Autodesk Inventor part; units mm, degrees
ref_plane "Płaszczyzna konstrukcyjna2" through (43, 47, -4.5) normal (0, 0, -1) x (-1, 0, 0)
ref_plane "YZ Plane" through (0, 0, 0) normal (1, 0, 0) x (0, 1, 0)
ref_plane "XZ Plane" through (0, 0, 0) normal (0, 1, 0) x (-1, 0, 0)
sketch "Szkic1" plane through (0, 0, 0) normal (0, 0, 1) x (1, 0, 0)
  line L0 (0, 0) -> (41, 0)
  line L1 (41, 0) -> (41, 45)
  line L2 (41, 45) -> (0, 45)
  line L3 (0, 45) -> (0, 0)
  line L4 (0, 45) -> (-2, 45)
  line L5 (-2, 45) -> (-2, 47)
  line L6 (41, 0) -> (41, -2)
  line L7 (41, -2) -> (43, -2)
  line L8 (43, -2) -> (-2, -2)
  line L9 (-2, -2) -> (-2, 47)
  line L10 (-2, 47) -> (43, 47)
  line L11 (43, 47) -> (43, -2)
  line L12 (41, 45) -> (37, 45)
  line L13 (37, 45) -> (37, 47)
  line L14 (43, 47) -> (37, 47)
  line L15 (41, 45) -> (41, 41)
  line L16 (41, 41) -> (43, 41)
  line L17 (43, 47) -> (43, 41)
  line L18 (43, 47) -> (37, 47)
  line L19 (20.5, 47) -> (20.5, -2)
  line L20 (-2, 22.5) -> (43, 22.5)
  line L21 (0, 45) -> (41, 45)
  line L22 (43, 47) -> (-2, 47)
  line L23 (-2, 47) -> (-2, -2)
  line L24 (4, 45) -> (4, 47)
  line L25 (0, 41) -> (-2, 41)
  line L26 (41, 0) -> (0, 0)
  line L27 (0, 0) -> (0, 45)
  line L28 (0, 0) -> (-2, 0)
  line L29 (-2, -2) -> (43, -2)
  line L30 (43, -2) -> (43, 47)
  line L31 (41, 4) -> (43, 4)
  line L32 (-2, -2) -> (-2, 47)
  line L33 (4, 0) -> (4, -2)
  line L34 (0, 0) -> (0, 4)
  line L35 (0, 4) -> (-2, 4)
  line L36 (41, 0) -> (37, 0)
  line L37 (37, 0) -> (37, -2)
  line L38 (37, -2) -> (43, -2)
  dimension "d0" = 41
  dimension "d1" = 45
  dimension "d2" = 2
  dimension "d3" = 2
  dimension "d4" = 2
  dimension "d5" = 2
  dimension "d6" = 4
  dimension "d7" = 4
  dimension "d8" = 4
  dimension "d9" = 4
sketch "Szkic1 outline for Wyciągnięcie proste1" plane through (0, 0, 0) normal (0, 0, 1) x (1, 0, 0)
  line L0 (41, 41) -> (43, 41)
  line L1 (41, 45) -> (41, 41)
  line L2 (37, 45) -> (41, 45)
  line L3 (37, 47) -> (37, 45)
  line L4 (43, 47) -> (37, 47)
  line L5 (43, 41) -> (43, 47)
  line L6 (43, 4) -> (41, 4)
  line L7 (41, 4) -> (41, 0)
  line L8 (41, 0) -> (37, 0)
  line L9 (37, 0) -> (37, -2)
  line L10 (37, -2) -> (43, -2)
  line L11 (43, -2) -> (43, 4)
  line L12 (0, 4) -> (-2, 4)
  line L13 (0, 0) -> (0, 4)
  line L14 (4, 0) -> (0, 0)
  line L15 (4, -2) -> (4, 0)
  line L16 (-2, -2) -> (4, -2)
  line L17 (-2, 4) -> (-2, -2)
  line L18 (4, 45) -> (4, 47)
  line L19 (4, 47) -> (-2, 47)
  line L20 (-2, 47) -> (-2, 41)
  line L21 (-2, 41) -> (0, 41)
  line L22 (0, 41) -> (0, 45)
  line L23 (0, 45) -> (4, 45)
extrude "Wyciągnięcie proste1" add sketch "Szkic1 outline for Wyciągnięcie proste1" along normal blind 20 draft -1
sketch "Szkic2" plane through (0, 0, 0) normal (0, 0, -1) x (-1, 0, 0)
  line L0 (-43, 41) -> (-43, 47)
  line L1 (2, 4) -> (2, -2)
  line L2 (-43, 47) -> (2, 47)
  line L3 (2, 47) -> (2, -2)
  line L4 (2, -2) -> (-43, -2)
  line L5 (-43, -2) -> (-43, 47)
  line L6 (-37, 45) -> (-41, 45)
  line L7 (0, 0) -> (-41, 0)
  line L8 (-41, 0) -> (-41, 45)
  line L9 (-41, 45) -> (0, 45)
  line L10 (0, 45) -> (0, 0)
extrude "Wyciągnięcie proste2" add sketch "Szkic2" against normal blind 3 draft -1
sketch "Szkic3" plane through (0, 0, 0) normal (0, 0, -1) x (-1, 0, 0)
  line L0 (2, -2) -> (1.650899, -1.650899)
  line L1 (-43, -2) -> (-43, 47)
  line L2 (2, -2) -> (-43, -2)
  line L3 (-43, -2) -> (-43, 47)
  line L4 (-43, 47) -> (2, 47)
  line L5 (2, 47) -> (2, -2)
  circle A0 centre (-20.5, 22.5) radius 2.85
  circle A1 centre (-20.5, 22.5) radius 2.8
  point P0 (0, 0)
  dimension "d14" = 5.7
  dimension "d21" = 5.6
extrude "Wyciągnięcie proste3" add sketch "Szkic3" along normal blind 8 contours L1 L4 L5 L2 | A0
ref_plane "Płaszczyzna konstrukcyjna2" through (43, 47, -4.5) normal (0, 0, -1) x (-1, 0, 0)
ref_plane "Płaszczyzna konstrukcyjna1" through (43, 47, -8) normal (0, 0, -1) x (-1, 0, 0)
sketch "Szkic4" plane through (43, 47, -4.5) normal (0, 0, -1) x (-1, 0, 0)
  circle A0 centre (22.5, -24.5) radius 2.85
  circle A1 centre (22.5, -24.5) radius 1.5
  circle A2 centre (22.5, -24.5) radius 2.85
  point P0 (43, -47)
  dimension "d18" = 3
extrude "Wyciągnięcie proste4" add sketch "Szkic4" along normal blind 1
sketch "Szkic5" plane through (20.5, 22.5, -5.5) normal (0, 0, -1) x (-1, 0, 0)
  circle A0 centre (0, 0) radius 2.8
  circle A1 centre (0, 0) radius 2.4
  point P0 (20.5, -22.5)
  dimension "d22" = 4.8
extrude "Wyciągnięcie proste5" add sketch "Szkic5" along normal blind 2.5
sketch "Szkic6" plane through (20.5, 22.5, -4.5) normal (0, 0, 1) x (1, 0, 0)
  circle A0 centre (0, 0) radius 1.5
  circle A1 centre (0, 0) radius 2.8
  point P0 (-20.5, -22.5)
extrude "Wyciągnięcie proste6" add sketch "Szkic6" along normal blind 2
sketch "Szkic7" plane through (20.5, 22.5, -5.5) normal (0, 0, -1) x (-1, 0, 0)
  circle A0 centre (0, 0) radius 1.5
  circle A1 centre (0, 0) radius 2.4
  point P0 (20.5, -22.5)
extrude "Wyciągnięcie proste7" cut sketch "Szkic7" against normal blind 1.5
sketch "Szkic8" plane through (20.5, 22.5, -2.5) normal (0, 0, 1) x (1, 0, 0)
  circle A0 centre (0, 0) radius 1.4
  circle A1 centre (0, 0) radius 1.5
  point P0 (-20.5, -22.5)
  dimension "d29" = 2.8
extrude "Wyciągnięcie proste8" add sketch "Szkic8" against normal blind 1.5
properties part number "Część5_Drukowanie 3D"
The listing builds one solid part. Answer for the finished solid, in the listing's coordinates (mm). A direction names the side the tool comes from. Coordinates: 2 decimals unless noted, no trailing zeros. Write each loop counter-clockwise with the first axis right and the second up, starting at its lowest first coordinate (ties: lowest second). Pieces come first, ordered by that corner, then holes. Notation, with made-up numbers: M -21.5,9.25 L -14.5,9.25 A34 cw -14.5,42.25 Z; hole C 12.5,64.25 d5. An arc over 180 degrees is marked long. Put each result on its own line as item: value. Start each with the question number.
1. Consider line 1 (Y direction, x = 20.5, z = -0.95); line 2 (X direction, y = 27.5, z = 2.25); line 3 (Y direction, x = 40.5, z = 0.75). Determine where each line is inside the solid, lowest interval first. Write a range as from..to.
2. Flat-ended cylindrical pins translate along their axes: P1, Ø0.6, axis at x = 41.5, y = 15.5, coming from the +Z side; P2, Ø6.5, axis at x = 20.5, y = 22.5, coming from the +Z side; P3, Ø4.5, axis at x = 20, y = 22.5, coming from the +Z side. Find the tip coordinate at first contact, or state that the pin passes through.
3. Which of the six approach directions +Z, -Z, +X, -X, +Y, -Y give full straight-line access (tool end or side, diameter ignored) to faces 5 (the cylindrical face through (19.39, 24.63, -5.97)), 6 (the flat face through (-2, 23, -4)), 7 (the flat face through (25, 23, 0))?
4. A cutting plane is placed at B-B on y = 22.5. Write down the section's boundary in (x, z).
5. A cutting plane is placed at A-A on x = 20.5. Write down the section's boundary in (y, z).
6. A cutting plane is placed at C-C on z = 1. Write down the section's boundary in (x, y), then the cut area to 3 significant figures.
7. For a pull along X with two mould halves and no side action, classify faces 1 (the flat face through (43, 22, -4)), 2 (the flat face through (21, -1, 3)), 3 (the flat face through (19, 22, -2.5)), 4 (the flat face through (42, 23, 3)) as pulls with the +X half, pulls with the -X half, needs draft (parallel to the pull), parting line crosses it, or undercut.
8. A cutting plane is placed at D-D on z = 9. Write down the section's boundary in (x, y), then the cut area to 3 significant figures.
Resolved:
1. line 1: y = -2..19.7, 25.3..47
1. line 2: x = -1.96..-0.04, 41.04..42.96
1. line 3: y = -1.99..-0.01, 45.01..46.99
2. P1: stops at z = 3
2. P2: stops at z = 0
2. P3: stops at z = -2.5
3. face 5: -Z
3. face 6: +Z, -Z, -X, +Y, -Y
3. face 7: +Z
4. outline: M -2,-8 L 18.1,-8 L 18.1,-4 L 19.1,-4 L 19.1,-2.5 L 17.7,-2.5 L 17.7,0 L 0,0 L -0.05,3 L -1.95,3 L -2,0 Z; M 21.9,-4 L 22.9,-4 L 22.9,-8 L 43,-8 L 43,0 L 42.95,3 L 41.05,3 L 41,0 L 23.3,0 L 23.3,-2.5 L 21.9,-2.5 Z
5. outline: M -2,-8 L 20.1,-8 L 20.1,-4 L 21.1,-4 L 21.1,-2.5 L 19.7,-2.5 L 19.7,0 L 0,0 L -0.05,3 L -1.95,3 L -2,0 Z; M 23.9,-4 L 24.9,-4 L 24.9,-8 L 47,-8 L 47,0 L 46.95,3 L 45.05,3 L 45,0 L 25.3,0 L 25.3,-2.5 L 23.9,-2.5 Z
6. outline: M -1.98,-1.98 L 42.98,-1.98 L 42.98,46.98 L -1.98,46.98 Z; hole M -0.02,-0.02 L 41.02,-0.02 L 41.02,45.02 L -0.02,45.02 Z
6. area: 354 mm2
7. face 1: pulls with the +X half
7. face 2: undercut
7. face 3: undercut
7. face 4: needs draft
8. outline: M -1.84,-1.84 L 3.84,-1.84 L 3.84,-0.16 L -0.16,-0.16 L -0.16,3.84 L -1.84,3.84 Z; M -1.84,41.16 L -0.16,41.16 L -0.16,45.16 L 3.84,45.16 L 3.84,46.84 L -1.84,46.84 Z; M 37.16,-1.84 L 42.84,-1.84 L 42.84,3.84 L 41.16,3.84 L 41.16,-0.16 L 37.16,-0.16 Z; M 37.16,45.16 L 41.16,45.16 L 41.16,41.16 L 42.84,41.16 L 42.84,46.84 L 37.16,46.84 Z
8. area: 65.3 mm2
